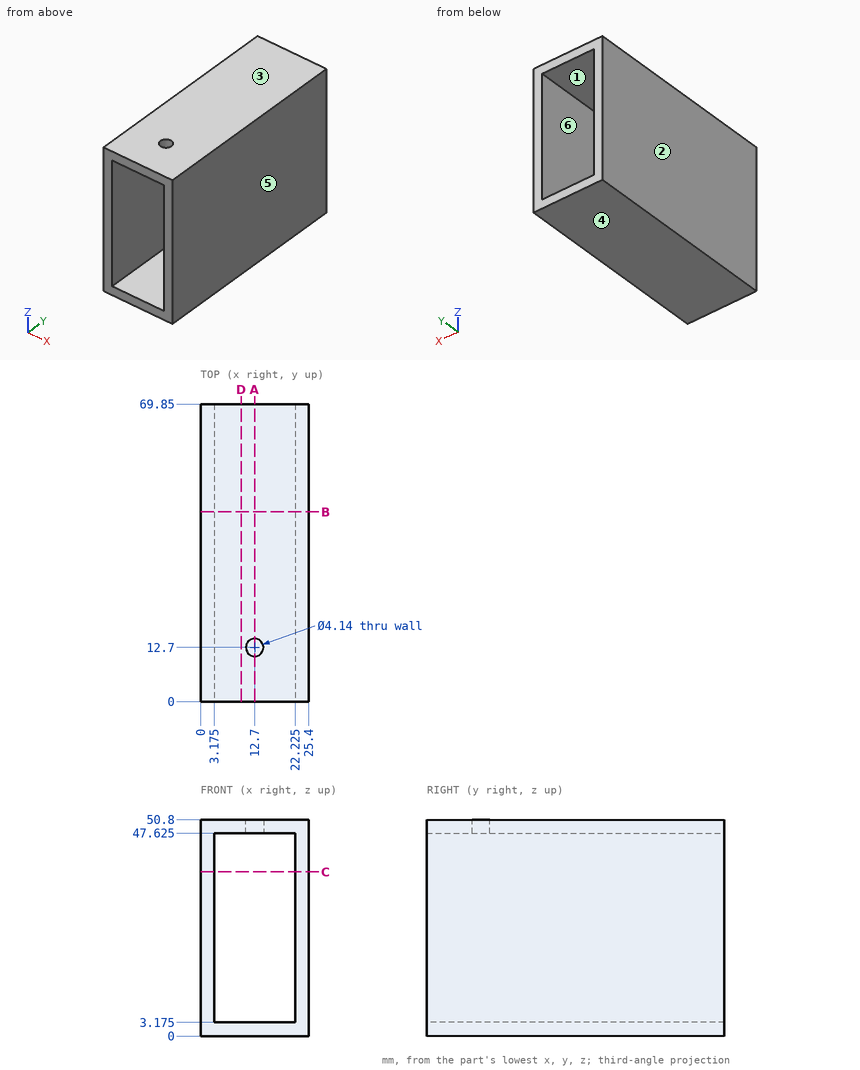
Study the drawing (mm; zero at the part's minimum x, y, z) and answer. A direction names the side the tool comes from. Give positions to 0.01 mm unless a question says otherwise; leave off trailing zeros. Order: outer loops, then holes, each group sorted by start corner. A loop starts at its lowest first (then second) coordinate and runs counter-clockwise, first axis right, second up. Notation, with made-up numbers: M -35.5,74.5 L 19.5,74.5 A32 ccw 19.5,102.5 Z; hole C -8.5,7.5 d4. An arc over 180 degrees is marked long. Put each result on its own line as item: value. Start each with the question number.
Item 1: Which of the six approach directions +Z, -Z, +X, -X, +Y, -Y give full straight-line access (tool end or side, diameter ignored) to the marked faces 5 and 6?
Item 2: Find the intervals of material crossed by line 1 along Z through (x, y) = (20.25, 38.5) (3 decimals); line 2 along Y through (x, z) = (12.7, 49.45); line 3 along X through (y, z) = (4, 30.5) (3 decimals), in increasing order.
Item 3: The part is cut by section A-A, the plane x = 12.7. State how many separate pieces and enclosed holes the cut face has.
Item 4: The part is cut by section D-D, the plane x = 9.5. Determine the outline of the cut face in (y, z) (3 decimals).
Item 5: For a pull along Z with two mould halves and no side action, classify the marked faces 1, 2, 3 and 4 as +Z half, -Z half, draft (parallel to the pull), parting line (faces both ways), or undercut.
Item 6: The part is cut by section C-C, the plane z = 38.5. Determine the outline of the cut face in (x, y) (3 decimals).
Item 7: The part is cut by section B-B, the plane y = 44.5. Determine the outline of the cut face in (x, z) (3 decimals).
Answer key:
1. face 5: +Z, -Z, +X, +Y, -Y
1. face 6: +Y, -Y
2. line 1: z = 0 to 3.175, 47.625 to 50.8
2. line 2: y = 0 to 10.63, 14.77 to 69.85
2. line 3: x = 0 to 3.175, 22.225 to 25.4
3. separate pieces: 3
3. enclosed holes: 0
4. outline: M 0,0 L 69.85,0 L 69.85,3.175 L 0,3.175 Z; M 0,47.625 L 69.85,47.625 L 69.85,50.8 L 0,50.8 Z
5. face 1: undercut
5. face 2: draft
5. face 3: +Z half
5. face 4: -Z half
6. outline: M 0,0 L 3.175,0 L 3.175,69.85 L 0,69.85 Z; M 22.225,0 L 25.4,0 L 25.4,69.85 L 22.225,69.85 Z
7. outline: M 0,0 L 25.4,0 L 25.4,50.8 L 0,50.8 Z; hole M 3.175,3.175 L 22.225,3.175 L 22.225,47.625 L 3.175,47.625 Z
